```python
from build123d import *

# Parameters (mm, degrees)
ESQUISSE1_W             = 130
ESQUISSE1_H             = 130
BOSS_EXTRU_1_DEPTH      = 3
CHANFREIN1_SIZE         = 3
ESQUISSE2_W             = 10
ESQUISSE2_H             = 5
BOSS_EXTRU_2_DEPTH      = 10
ESQUISSE4_R             = 1.75
ENL_V_MAT_EXTRU_1_DEPTH = 175.051716452
ESQUISSE5_R             = 1.75
ENL_V_MAT_EXTRU_2_DEPTH = 171.724954239


with BuildPart() as part:
    # Esquisse1 → Boss.-Extru.1 (new body)
    with BuildSketch(Plane.XY):
        with Locations((65, 65)):
            Rectangle(ESQUISSE1_W, ESQUISSE1_H)
    extrude(amount=BOSS_EXTRU_1_DEPTH)

    # Chanfrein1
    chanfrein1_edges = [part.edges().sort_by_distance(p)[0] for p in [
        (65, 130, 0),
        (130, 65, 0),
        (65, 0, 0),
        (0, 65, 0),
    ]]
    chamfer(chanfrein1_edges, length=CHANFREIN1_SIZE - 0.0001)  # a hair under: the kernel refuses the full size

    # Esquisse2 → Boss.-Extru.2 (add)
    with BuildSketch(Plane.XY.offset(3)):
        with Locations((5, 107.4)):
            Rectangle(ESQUISSE2_W, ESQUISSE2_H)
        with Locations((5, 17.5)):
            Rectangle(ESQUISSE2_W, ESQUISSE2_H)
        with Locations((125, 22.6)):
            Rectangle(ESQUISSE2_W, ESQUISSE2_H)
        with Locations((125, 112.5)):
            Rectangle(ESQUISSE2_W, ESQUISSE2_H)
    extrude(amount=BOSS_EXTRU_2_DEPTH)

    # Esquisse4 → Enlèv. mat.-Extru.1 (cut, through all)
    with BuildSketch(Plane.XZ.offset(-15)):
        with Locations(Location((5, 8, 0), (0, 0, 270))):
            Circle(ESQUISSE4_R)
    extrude(amount=-ENL_V_MAT_EXTRU_1_DEPTH, mode=Mode.SUBTRACT)

    # Esquisse5 → Enlèv. mat.-Extru.2 (cut, through all)
    with BuildSketch(Plane.XZ.offset(-20.1)):
        with Locations(Location((125, 8, 0), (0, 0, 270))):
            Circle(ESQUISSE5_R)
    extrude(amount=-ENL_V_MAT_EXTRU_2_DEPTH, mode=Mode.SUBTRACT)


solid = part.part
```
Geometry check sheet. Reference: the model listing, model coordinates, mm. A direction names the side the tool comes from. Give positions to 0.01 mm unless a question says otherwise; leave off trailing zeros. Use one line per item in the form item = value.
Item 1: Access from +Z, -Z, +X, -X, +Y, -Y to the whole of each face (thin tool, end or side, straight path). Record for faces 4 (the flat face through (10, 17, 8)), 5 (the flat face through (7, 104.9, 8)), 6 (the flat face through (120, 23, 8)), 7 (the flat face through (125, 23, 13)).
Results list:
face_4 = +Z, +X, +Y, -Y
face_5 = +Z, +X, -X
face_6 = +Z, -X, +Y, -Y
face_7 = +Z, +X, -X, +Y, -Y
Item 2: Mould release check, pull along Y, two halves, no side actions. Record for faces 1 (the cylindrical face through (123.29, 112.46, 8.38)), 2 (the flat face through (123, 20.1, 8)), 3 (the flat face through (123, 25.1, 8)): released by +Y, released by -Y, zero draft, split by the parting line, or undercut.
Results list:
face_1 = zero draft
face_2 = released by -Y
face_3 = undercut
Item 3: Scan lines: line 1 (X direction, y = 108, z = 8); line 2 (Z direction, x = 72, y = 63.5); line 3 (X direction, y = 24.5, z = 5.75). Record each from-to range of solid material in increasing order.
Results list:
line_1 = 0 to 3.25, 6.75 to 10
line_2 = 0 to 3
line_3 = 120 to 130
Item 4: Depth check by flat-ended pin: pin 1 Ø4 at (y, z) = (18, 8) entering from +X; pin 2 Ø5 at (x, z) = (3.5, 9) entering from -Y; pin 3 Ø2 at (x, y) = (37.5, 82.5) entering from +Z; pin 4 Ø5 at (y, z) = (104.5, 9.5) entering from -X. Enter the tip coordinate at first touch or a pass-through.
Results list:
pin_1 = 10
pin_2 = 15
pin_3 = 3
pin_4 = 0
Item 5: Sectioned sample at A-A on z = 8. Count the separate pieces of the cut face and the enclosed holes in it, plus the area to 3 significant figures.
Results list:
separate_pieces = 8
enclosed_holes = 0
area = 130 mm2
